Part model, mm, in its own coordinate system. A direction names the side the tool comes from. Give positions to 0.01 mm unless a question says otherwise; leave off trailing zeros. Loops run counter-clockwise (first coordinate to the right, second up) from the corner with the lowest first, then second, coordinate; pieces in that order, holes last. Notation, with made-up numbers: (44, -19) -> (85, -19) arc R23 cw to (85, 15) -> close; hole circle Ø7 at (35.5, -15.75). An arc over 180 degrees is marked (long way). One line per question, with ' | ' between items.
```python
from build123d import *

# Parameters (mm, degrees)
SKETCH_1_W               = 75
SKETCH_1_H               = 40
EXTRUDE_1_DEPTH          = 10
SKETCH_2_W               = 75
SKETCH_2_H               = 40
SKETCH_2_W_2             = 65
SKETCH_2_H_2             = 30
EXTRUDE_2_DEPTH          = 30
FILLET_2_R               = 2
SKETCH_3_W               = 5
SKETCH_3_H               = 5
CUT_EXTRUDE_1_DEPTH      = 30
EXTRUDE_3_REACH          = 72.682
SKETCH_4_W               = 40
SKETCH_4_H               = 69.781317598
SKETCH_5_W               = 69.781317598
SKETCH_5_H               = 40
EXTRUDE_4_DEPTH          = 45
CUT_EXTRUDE_2_DEPTH      = 109.313665007
CUT_EXTRUDE_3_DEPTH      = 93.843161337
CUT_EXTRUDE_3_DEPTH_BACK = 93.843161337
SKETCH_9_R               = 2.5
CUT_EXTRUDE_4_DEPTH      = 93.843161337
CUT_EXTRUDE_4_DEPTH_BACK = 93.843161337
FILLET_3_R               = 4
SKETCH_14_W              = 25
SKETCH_14_H              = 5
CUT_EXTRUDE_5_DEPTH      = 30


with BuildPart() as part:
    # 草图1 → 凸台-拉伸1 (new body)
    with BuildSketch(Plane(origin=(0, 0, 0), x_dir=(1, 0, 0), z_dir=(0, 1, 0))):
        Rectangle(SKETCH_1_W, SKETCH_1_H)
    extrude(amount=EXTRUDE_1_DEPTH)

    # 草图2 → 凸台-拉伸2 (add)
    with BuildSketch(Plane(origin=(0, 10, 0), x_dir=(1, 0, 0), z_dir=(0, 1, 0))):
        Rectangle(SKETCH_2_W, SKETCH_2_H)
        Rectangle(SKETCH_2_W_2, SKETCH_2_H_2, mode=Mode.SUBTRACT)
    extrude(amount=EXTRUDE_2_DEPTH)

    # 圆角2
    fillet_2_edges = [part.edges().sort_by_distance(p)[0] for p in [
        (32.5, 25, -15),
        (-32.5, 25, -15),
        (-32.5, 25, 15),
        (32.5, 25, 15),
    ]]
    fillet(fillet_2_edges, radius=FILLET_2_R)

    # 草图3 → 切除-拉伸1 (cut)
    with BuildSketch(Plane(origin=(0, 40, 0), x_dir=(1, 0, 0), z_dir=(0, 1, 0))):
        with Locations((-35, -2.5)):
            Rectangle(SKETCH_3_W, SKETCH_3_H)
        with Locations((-35, 2.5)):
            Rectangle(SKETCH_3_W, SKETCH_3_H)
        with Locations((35, -2.5)):
            Rectangle(SKETCH_3_W, SKETCH_3_H)
        with Locations((35, 2.5)):
            Rectangle(SKETCH_3_W, SKETCH_3_H)
    extrude(amount=-CUT_EXTRUDE_1_DEPTH, mode=Mode.SUBTRACT)

    # 凸台-拉伸3: up to this face of the body (flat: up to its plane)
    extrude_3_end = Plane(part.part.faces().sort_by_distance((0, 0, 0))[0])
    # 草图4 → 凸台-拉伸3 (add, up to the picked face)
    with BuildSketch(Plane(origin=(5.037118095, -12.787469251, 0), x_dir=(0, 0, -1), z_dir=(0.3665012267242981, -0.9304175679820242, 0)), mode=Mode.PRIVATE) as extrude_3_sk1:
        Rectangle(SKETCH_4_W, SKETCH_4_H)
    extrude_3_tool1 = split(extrude(extrude_3_sk1.sketch, amount=-EXTRUDE_3_REACH, mode=Mode.PRIVATE), bisect_by=extrude_3_end, keep=Keep.BOTH, mode=Mode.PRIVATE)
    add(extrude_3_tool1.solids().sort_by(Axis((5.037118, -12.787469, 0), (-0.3665012267242981, 0.9304175679820242, 0)))[0])

    # 草图5 → 凸台-拉伸4 (add)
    with BuildSketch(Plane(origin=(5.037118095, -12.787469251, 0), x_dir=(0.9304175679820242, 0.36650122672429813, 0), z_dir=(0.36650122672429813, -0.9304175679820244, 0))):
        Rectangle(SKETCH_5_W, SKETCH_5_H)
    extrude(amount=EXTRUDE_4_DEPTH)

    # 草图7 → 切除-拉伸2 (cut, through all)
    with BuildSketch(Plane(origin=(32.462881905, 12.787469251, 0), x_dir=(0, 0, -1), z_dir=(0.9304175679820242, 0.3665012267242982, 0))):
        with BuildLine():
            ThreePointArc((14, -28.743796002), (0, -14.743796002), (-14, -28.743796002))
            Line((-14, -28.743796002), (-14, -58.743796002))
            Line((-14, -58.743796002), (14, -58.743796002))
            Line((14, -58.743796002), (14, -28.743796002))
        make_face()
    extrude(amount=-CUT_EXTRUDE_2_DEPTH, mode=Mode.SUBTRACT)

    # 草图9 → 切除-拉伸3 (cut, two sides: drawn at the far end of the back side and taken through both)
    with BuildSketch(Plane.XY.offset(-14).offset(-CUT_EXTRUDE_3_DEPTH_BACK)):
        with Locations((-1.924711649, -49.385573493)):
            Circle(SKETCH_9_R)
        with Locations((35.088525122, -34.805671792)):
            Circle(SKETCH_9_R)
    extrude(amount=CUT_EXTRUDE_3_DEPTH + CUT_EXTRUDE_3_DEPTH_BACK, mode=Mode.SUBTRACT)

    # 草图11 → 切除-拉伸4 (cut, two sides: drawn at the far end of the back side and taken through both)
    with BuildSketch(Plane.XY.offset(-14).offset(-CUT_EXTRUDE_4_DEPTH_BACK)):
        with BuildLine():
            Line((5.98428163, -28.53616522), (12.031551871, -43.888055092))
            ThreePointArc((12.031551871, -43.888055092), (12.812044317, -46.587712953), (13.075288351, -49.385573493))
            ThreePointArc((13.075288351, -49.385573493), (12.047893904, -54.84142302), (9.106449143, -59.549897946))
            Line((9.106449143, -59.549897946), (33.952897452, -49.762621675))
            ThreePointArc((33.952897452, -49.762621675), (26.182824368, -46.875820676), (21.132261602, -40.303190193))
            Line((21.132261602, -40.303190193), (15.084991361, -24.951300321))
            Line((15.084991361, -24.951300321), (5.98428163, -28.53616522))
        make_face()
        with BuildLine():
            ThreePointArc((-3.06033932, -64.342523376), (-10.830412504, -61.455722303), (-15.880975261, -54.883091661))
            Line((-15.880975261, -54.883091661), (-10.933208608, -67.443729062))
            Line((-10.933208608, -67.443729062), (-3.06033932, -64.342523376))
        make_face()
        with BuildLine():
            Line((53.992555203, -41.868790559), (49.044788748, -29.308153662))
            ThreePointArc((49.044788748, -29.308153662), (49.825281115, -32.007811395), (50.088525122, -34.805671792))
            ThreePointArc((50.088525122, -34.805671792), (49.061130675, -40.261521319), (46.119685914, -44.969996245))
            Line((46.119685914, -44.969996245), (53.992555203, -41.868790559))
        make_face()
    extrude(amount=CUT_EXTRUDE_4_DEPTH + CUT_EXTRUDE_4_DEPTH_BACK, mode=Mode.SUBTRACT)

    # 圆角3
    fillet_3_edges = [part.edges().sort_by_distance(p)[0] for p in [
        (5.98428163, -28.53616522, 17),
        (5.98428163, -28.53616522, -17),
        (15.084991361, -24.951300321, 17),
        (15.084991361, -24.951300321, -17),
    ]]
    fillet(fillet_3_edges, radius=FILLET_3_R)

    # 草图14 → 切除-拉伸5 (cut)
    with BuildSketch(Plane(origin=(0, 40, 0), x_dir=(1, 0, 0), z_dir=(0, 1, 0))):
        with Locations((0, -17.5)):
            Rectangle(SKETCH_14_W, SKETCH_14_H)
    cut_extrude_5 = extrude(amount=-CUT_EXTRUDE_5_DEPTH, mode=Mode.SUBTRACT)

    # 镜向1: 切除-拉伸5 across plane
    add(cut_extrude_5.mirror(Plane.XY), mode=Mode.SUBTRACT)


solid = part.part
```
1) Saw through at A-A (y = 25.5). Give the cut face in (x, z), and give its area (3 significant figures).
Found:
outline: (-37.5, -20) -> (-12.5, -20) -> (-12.5, -15) -> (-30.5, -15) arc R2 cw to (-32.5, -13) -> (-32.5, -5) -> (-37.5, -5) -> close; (-37.5, 5) -> (-32.5, 5) -> (-32.5, 13) arc R2 cw to (-30.5, 15) -> (-12.5, 15) -> (-12.5, 20) -> (-37.5, 20) -> close; (12.5, -20) -> (37.5, -20) -> (37.5, -5) -> (32.5, -5) -> (32.5, -13) arc R2 cw to (30.5, -15) -> (12.5, -15) -> close; (12.5, 15) -> (30.5, 15) arc R2 cw to (32.5, 13) -> (32.5, 5) -> (37.5, 5) -> (37.5, 20) -> (12.5, 20) -> close | area: 703 mm2
2) Tool access for faces 3 (the flat face through (-12.5, 25, -18)), 4 (the flat face through (0, -47, -14)), 5 (the cylindrical face through (14.38, -26.45, -16.96)), 6 (the flat face through (37.5, 20, 9)): list every direction of +Z, -Z, +X, -X, +Y, -Y with a clear straight run to the whole face (end or side of a thin tool).
Found:
face 3: +Z, -Z, +Y | face 4: +X, -Y | face 5: +Z, -Z | face 6: +Z, -Z, +X, +Y
3) Saw through at D-D (z = 0.5). Give the cut face in (x, y), and give its area (3 significant figures).
Found:
outline: (-37.5, 0) -> (-27.06, -26.51) -> (37.87, -0.94) -> (37.5, 0) -> (37.5, 10) -> (-37.5, 10) -> close | area: 1,780 mm2
4) Saw through at B-B (z = -9.5). Give the cut face in (x, y).
Found:
outline: (-37.5, 0) -> (-25.7, -29.96) -> (39.23, -4.39) -> (37.5, 0) -> (37.5, 40) -> (32.5, 40) -> (32.5, 10) -> (-32.5, 10) -> (-32.5, 40) -> (-37.5, 40) -> close
5) Drill centre lines: line 1 (Z direction, x = 24, y = 22.5); line 2 (Z direction, x = 46, y = -22.5); line 3 (X direction, y = 5, z = 11). Where is each one in solid material? Low to high.
Found:
line 1: -20 to -15, 15 to 20 | line 2: -20 to -14, 14 to 20 | line 3: -37.5 to 37.5
6) Saw through at C-C (x = 36). State how many separate pieces and enclosed holes the cut face has, and give its area (3 significant figures).
Found:
separate pieces: 3 | enclosed holes: 0 | area: 1,970 mm2
7) Pin check, flat tips, straight feed: P1, Ø4, axis at y = 26.5, z = 11, coming from the +X side; P2, Ø4, axis at y = -49.5, z = 10.5, coming from the -X side; P3, Ø6.5, axis at x = -1.92, y = -49.39, coming from the +Z side; P4, Ø10, axis at x = 15, z = -4, coming from the -Y side. Stop position of each tip, or through.
Found:
P1: x = 37.5 | P2: through | P3: z = 20 | P4: y = -13.89
8) Pull direction Z, two halves, no side cores. Call faces 1 (the flat face through (-32.5, 25, -9)), 2 (the cylindrical face through (26.278, -46.945, -17.042)): pulls with the +Z half, pulls with the -Z half, needs draft (parallel to the pull), parting line crosses it, or undercut.
Found:
face 1: undercut | face 2: needs draft
